from build123d import *

# Parameters (mm, degrees)
F3_SIZE  = 0.5
F4_SIZE2 = 0.5
F4_SIZE  = 0.5


with BuildPart() as f2:
    # F0 (on Front) → F2 (revolve)
    with BuildSketch(Plane.XZ):
        with BuildLine():
            Line((26.5, -9.875), (26.5, 9.875))
            Line((26.5, 9.875), (-26.5, 9.875))
            Line((-26.5, 9.875), (-26.5, -9.875))
            Line((-26.5, -9.875), (-22.5, -9.875))
            ThreePointArc((-22.5, -9.875), (0, -4.8510921188), (22.5, -9.875))
            Line((22.5, -9.875), (26.5, -9.875))
        make_face()
    revolve(axis=Axis((0, 0, 15.125), (1, 0, 0)))

    # F3
    f3_edges = [f2.edges().sort_by_distance(p)[0] for p in [
        (26.5, 0, 40.125),
        (-26.5, 0, 40.125),
    ]]
    chamfer(f3_edges, length=F3_SIZE)

    # F4
    f4_edges = [f2.edges().sort_by_distance(p)[0] for p in [
        (26.5, 0, 20.375),
        (-26.5, 0, 20.375),
    ]]
    chamfer(f4_edges, length=F4_SIZE, length2=F4_SIZE2)


solid = f2.part
Source: CAD feature listing. Evaluate the final solid. Frame: model axes, mm. Round coordinates to 2 decimals unless told otherwise and drop trailing zeros. Loops run counter-clockwise (first coordinate to the right, second up) from the corner with the lowest first, then second, coordinate; pieces in that order, holes last. Notation, with made-up numbers: (-28.75, -4.75) - (11.25, -4.75) arc R25 cw to (11.25, 17.25) - close; hole circle Ø6 at (44, 82). An arc over 180 degrees is marked (long way). Write item = value, one per line. Start each with the question number.
Item 1: Material intervals for line 1 (Y direction, x = -13, z = 11); line 2 (Z direction, x = -4, y = 3.5); line 3 (Z direction, x = 13, y = -2.5), sorted ascending.
Item 2: Section query C-C on x = 20.5. Output: boundary loops of the cut face in (y, z) (3 decimals).
Item 3: Section query B-B on x = -3. Output: boundary loops of the cut face in (y, z) (3 decimals).
Item 4: Section query A-A on y = 0. Output: boundary loops of the cut face in (x, z) (3 decimals), plus the area to 3 significant figures.
Item 5: Mould query, pull axis Y, two halves, no side actions, for faces 1 (the face through (26.5, 6, 15)), 2 (the face through (24.274, -15.212, 34.964)), 3 (the face through (-0.36, 0.23, 20.37)). Classes: released by +Y, released by -Y, zero draft, split by the parting line, or undercut.
Item 6: First-contact query: pin 1 Ø6 at (x, y) = (9, 7.5) entering from -Z; pin 2 Ø6 at (x, z) = (15.5, -3.5) entering from +Y; pin 3 Ø5 at (x, z) = (10, 16.5) entering from -Y; pin 4 Ø17 at (y, z) = (0, 15.125) entering from -X. Flat tips, straight axial feed; report the tip coordinate or a pass-through.
Results list:
q1.line_1 = -21.2 to -3.25, 3.25 to 21.2
q1.line_2 = -4.7 to 11.21, 19.04 to 34.95
q1.line_3 = -6.33 to 10.51, 19.74 to 36.58
q2.outline = circle Ø48.22 at (0, 15.125); hole circle Ø10.5 at (0, 15.125)
q3.outline = circle Ø40.122 at (0, 15.125); hole circle Ø10.5 at (0, 15.125)
q4.outline = (-26.5, -9.375) - (-26, -9.875) - (-22.5, -9.875) arc R52.896 cw to (22.5, -9.875) - (26, -9.875) - (26.5, -9.375) - (26.5, 9.375) - (26, 9.875) - (-26, 9.875) - (-26.5, 9.375) - close; (-26.5, 20.875) - (-26, 20.375) - (26, 20.375) - (26.5, 20.875) - (26.5, 39.625) - (26, 40.125) - (22.5, 40.125) arc R52.896 cw to (-22.5, 40.125) - (-26, 40.125) - (-26.5, 39.625) - close
q4.area = 1,790 mm²
q5.face_1 = zero draft
q5.face_2 = split by the parting line
q5.face_3 = undercut
q6.pin_1 = -5.34
q6.pin_2 = 16.2
q6.pin_3 = -21.44
q6.pin_4 = -26.5
